from build123d import *

# Parameters (mm, degrees)
ESQUISSE1_R             = 2
BOSS_EXTRU_1_DEPTH      = 15
ESQUISSE3_W             = 38
ESQUISSE3_H             = 20
BOSS_EXTRU_2_DEPTH      = 8
ESQUISSE4_R             = 3.2
ENL_V_MAT_EXTRU_1_DEPTH = 10
ESQUISSE1_3_R           = 2
ENL_V_MAT_EXTRU_3_DEPTH = 15


with BuildPart() as part:
    # Esquisse1 → Boss.-Extru.1 (new body)
    # profile 1 of 4: a face of its own
    with BuildSketch(Plane(origin=(0, 0, 0), x_dir=(1, 0, 0), z_dir=(0, 1, 0))):
        Polygon((11, -10), (11, 0), (11, 10), (19, 10), (19, -10), align=None)
        with Locations((15, 0)):
            Circle(ESQUISSE1_R, mode=Mode.SUBTRACT)
    # profile 2 of 4: a face of its own
    with BuildSketch(Plane(origin=(0, 0, 0), x_dir=(1, 0, 0), z_dir=(0, 1, 0))):
        with Locations((15, 0)):
            Circle(ESQUISSE1_R)
    # profile 3 of 4: a face of its own
    with BuildSketch(Plane(origin=(0, 0, 0), x_dir=(1, 0, 0), z_dir=(0, 1, 0))):
        Polygon((-19, -10), (-11, -10), (-11, 0), (-11, 10), (-19, 10), align=None)
        with Locations((-15, 0)):
            Circle(ESQUISSE1_R, mode=Mode.SUBTRACT)
    # profile 4 of 4: a face of its own
    with BuildSketch(Plane(origin=(0, 0, 0), x_dir=(1, 0, 0), z_dir=(0, 1, 0))):
        with Locations((-15, 0)):
            Circle(ESQUISSE1_R)
    extrude(amount=BOSS_EXTRU_1_DEPTH)

    # Esquisse3 → Boss.-Extru.2 (add)
    with BuildSketch(Plane(origin=(0, 15, 0), x_dir=(1, 0, 0), z_dir=(0, 1, 0))):
        Rectangle(ESQUISSE3_W, ESQUISSE3_H)
    extrude(amount=BOSS_EXTRU_2_DEPTH)

    # Esquisse4 → Enl_v. mat.-Extru.1 (cut)
    with BuildSketch(Plane(origin=(0, 23, 0), x_dir=(1, 0, 0), z_dir=(0, 1, 0))):
        with Locations(Location((0, 0, 0), (0, 0, 270))):
            Circle(ESQUISSE4_R)
    extrude(amount=-ENL_V_MAT_EXTRU_1_DEPTH, mode=Mode.SUBTRACT)

    # Esquisse1_3 → Enl_v. mat.-Extru.3 (cut)
    with BuildSketch(Plane(origin=(0, 0, 0), x_dir=(1, 0, 0), z_dir=(0, 1, 0))):
        with Locations(Location((-15, 0, 0), (0, 0, 270))):
            Circle(ESQUISSE1_3_R)
        with Locations(Location((15, 0, 0), (0, 0, 270))):
            Circle(ESQUISSE1_3_R)
    extrude(amount=ENL_V_MAT_EXTRU_3_DEPTH, mode=Mode.SUBTRACT)


solid = part.part
Build history of the part. All positions in model axes, mm. A direction names the side the tool comes from. Coordinates: 2 decimals unless noted, no trailing zeros. Order: outer loops, then holes, each group sorted by start corner. A loop starts at its lowest first (then second) coordinate and runs counter-clockwise, first axis right, second up. Notation, with made-up numbers: (8, 15) -> (67, 15) arc R26 cw to (67, 48) -> close; hole circle Ø9 at (-26.75, 43). An arc over 180 degrees is marked (long way). One line per item, written item: value.
(1) Slice it at B-B, the plane x = 0. List the corners of the cut face in (y, z).
Checked values:
outline: (15, -10) -> (23, -10) -> (23, -3.2) -> (15, -3.2) -> close; (15, 3.2) -> (23, 3.2) -> (23, 10) -> (15, 10) -> close
(2) Slice it at A-A, the plane y = 5.5. List the corners of the cut face in (x, z), plus the area to 3 significant figures.
Checked values:
outline: (-19, -10) -> (-11, -10) -> (-11, 10) -> (-19, 10) -> close; (11, -10) -> (19, -10) -> (19, 10) -> (11, 10) -> close; hole circle Ø4 at (-15, 0); hole circle Ø4 at (15, 0)
area: 295 mm2
(3) Mould opens along X. For faces 4 (the flat face through (0, 16, -10)), 5 (the flat face through (-19, 11, 0)), 6 (the flat face through (11, 7, 0)), 7 (the flat face through (19, 11, 0)) say: pulls with the +X half, pulls with the -X half, needs draft (parallel to the pull), parting line crosses it, or undercut.
Checked values:
face 4: needs draft
face 5: pulls with the -X half
face 6: undercut
face 7: pulls with the +X half
(4) Slice it at D-D, the plane z = 8. List the corners of the cut face in (x, y), plus the area to 3 significant figures.
Checked values:
outline: (-19, 0) -> (-11, 0) -> (-11, 15) -> (11, 15) -> (11, 0) -> (19, 0) -> (19, 23) -> (-19, 23) -> close
area: 544 mm2
(5) Tool access for faces 1 (the flat face through (-4, 23, 0)), 2 (the flat face through (-11, 7, 0)), 3 (the flat face through (15, 15, 0)): list every direction of +Z, -Z, +X, -X, +Y, -Y with a clear straight run to the whole face (end or side of a thin tool).
Checked values:
face 1: +Z, -Z, +X, -X, +Y
face 2: +Z, -Z, -Y
face 3: -Y
(6) Slice it at C-C, the plane z = 0. List the corners of the cut face in (x, y).
Checked values:
outline: (-19, 0) -> (-17, 0) -> (-17, 15) -> (-13, 15) -> (-13, 0) -> (-11, 0) -> (-11, 15) -> (-3.2, 15) -> (-3.2, 23) -> (-19, 23) -> close; (3.2, 15) -> (11, 15) -> (11, 0) -> (13, 0) -> (13, 15) -> (17, 15) -> (17, 0) -> (19, 0) -> (19, 23) -> (3.2, 23) -> close
(7) Probe line 1 (X direction, y = 10, z = 0); line 2 (X direction, y = 21.5, z = 0); line 3 (Y direction, x = 9, z = -2). List the from-to ranges inside material, lowest first. Write a range as [from, to].
Checked values:
line 1: [-19, -17], [-13, -11], [11, 13], [17, 19]
line 2: [-19, -3.2], [3.2, 19]
line 3: [15, 23]
(8) Drop flat-ended pins along their axis: pin 1 Ø4.5 at (x, z) = (15, 0) entering from -Y; pin 2 Ø6 at (x, z) = (5.5, 0.5) entering from -Y. Give the stop position or say it passes through.
Checked values:
pin 1: y = 0
pin 2: y = 15
